The figure shows three views and two pictorial views of one solid part (mm, origin at its lowest corner). Answer the questions. A direction names the side the tool comes from. Give positions to 0.01 mm unless a question says otherwise; leave off trailing zeros. Write each loop counter-clockwise with the first axis right and the second up, starting at its lowest first coordinate (ties: lowest second). Pieces come first, ordered by that corner, then holes. Notation, with made-up numbers: M 71.25,33 L 124.25,33 A15 cw 124.25,45 Z; hole C 54,-29 d7. An arc over 180 degrees is marked long. Return JSON: item names as keys, results as strings.
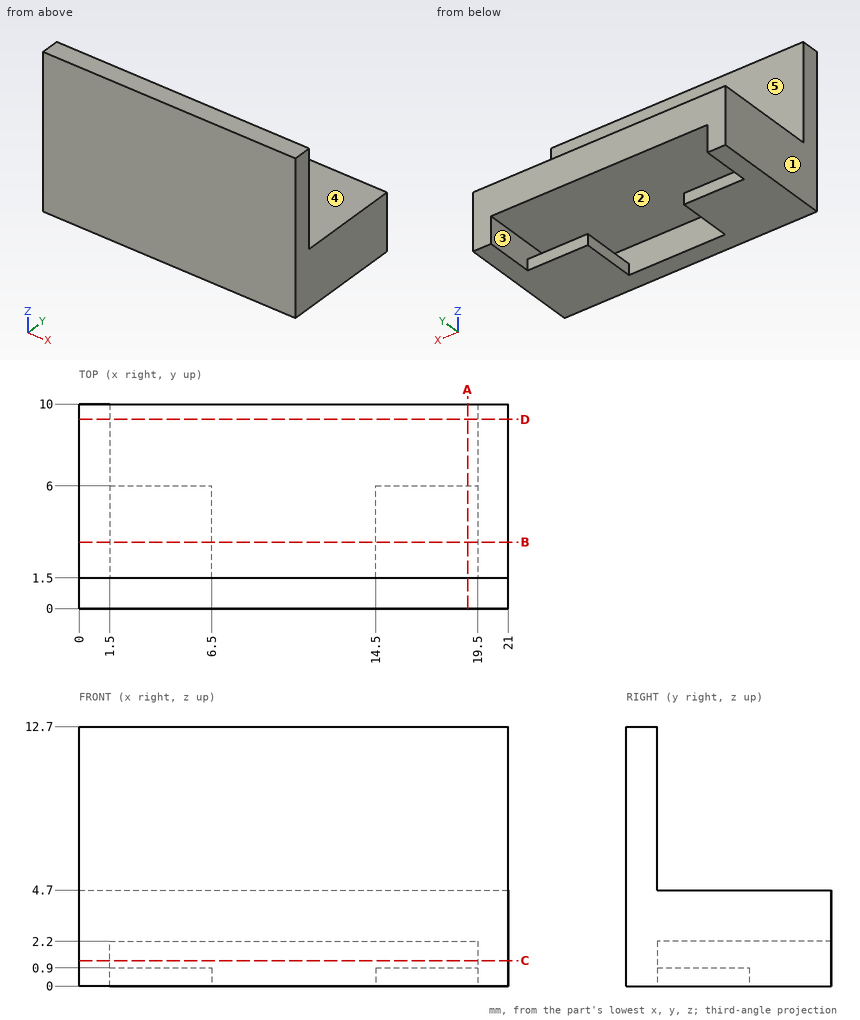
Item 1: Given pin 1 Ø0.7 at (x, z) = (6.5, 1) entering from +Y; pin 2 Ø3.5 at (x, y) = (17.5, 4) entering from +Z; pin 3 Ø4 at (x, z) = (7, 8) entering from +Y; pin 4 Ø5 at (x, z) = (3, 3) entering from -Y, each flat-ended and moving along its own axis, determine where each tip first touches the part or whether it passes through.
Geometry results:
{"pin 1": "stops at y = 6", "pin 2": "stops at z = 4.7", "pin 3": "stops at y = 1.5", "pin 4": "stops at y = 0"}
Item 2: A cutting plane is placed at B-B, the plane y = 3.25. Write down the section's boundary in (x, z).
Geometry results:
{"outline": "M 0,0 L 6.5,0 L 6.5,0.9 L 1.5,0.9 L 1.5,2.2 L 19.5,2.2 L 19.5,0.9 L 14.5,0.9 L 14.5,0 L 21,0 L 21,4.7 L 0,4.7 Z"}
Item 3: A cutting plane is placed at C-C, the plane z = 1.25. Write down the section's boundary in (x, y), plus the area to 3 significant figures.
Geometry results:
{"outline": "M 0,0 L 21,0 L 21,10 L 19.5,10 L 19.5,1.5 L 1.5,1.5 L 1.5,10 L 0,10 Z", "area": "57.0 mm2"}
Item 4: Which of the six approach directions +Z, -Z, +X, -X, +Y, -Y give full straight-line access (tool end or side, diameter ignored) to the marked faces 1 and 2?
Geometry results:
{"face 1": "+Z, -Z, -X, +Y, -Y", "face 2": "+Y"}
Item 5: A cutting plane is placed at D-D, the plane y = 9.25. Write down the section's boundary in (x, z).
Geometry results:
{"outline": "M 0,0 L 1.5,0 L 1.5,2.2 L 19.5,2.2 L 19.5,0 L 21,0 L 21,4.7 L 0,4.7 Z"}
Item 6: Find the intervals of material crossed by line 1 (X direction, y = 6.25, z = 1.5); line 2 (Z direction, x = 18.25, y = 2.5); line 3 (Z direction, x = 8.25, y = 5.5), in increasing order.
Geometry results:
{"line 1": "x = 0 to 1.5, 19.5 to 21", "line 2": "z = 0 to 0.9, 2.2 to 4.7", "line 3": "z = 2.2 to 4.7"}
Item 7: A cutting plane is placed at A-A, the plane x = 19. Write down the section's boundary in (y, z), plus the area to 4 significant figures.
Geometry results:
{"outline": "M 0,0 L 6,0 L 6,0.9 L 1.5,0.9 L 1.5,2.2 L 10,2.2 L 10,4.7 L 1.5,4.7 L 1.5,12.7 L 0,12.7 Z", "area": "44.35 mm2"}
Item 8: Determine the mould class of the marked faces 3, 4 and 5 for opening direction Z: +Z half, -Z half, draft (parallel to the pull), parting line (faces both ways), or undercut.
Geometry results:
{"face 3": "undercut", "face 4": "+Z half", "face 5": "draft"}
